Design review of the part built by this model. Coordinates are the model's own, in mm. A direction names the side the tool comes from. Round coordinates to 2 decimals unless told otherwise and drop trailing zeros. Loops run counter-clockwise (first coordinate to the right, second up) from the corner with the lowest first, then second, coordinate; pieces in that order, holes last. Notation, with made-up numbers: (63.5, 63) -> (72.5, 63) arc R11 ccw to (72.5, 76) -> close; hole circle Ø4 at (38.25, 79). An arc over 180 degrees is marked (long way). Answer as CSV lines item,"result". Start each with the question number.
(1) To check wall thickness, follow line 1 (Z direction, x = 45.5, y = -1.6); line 2 (Z direction, x = 25, y = -12); line 3 (X direction, y = -13, z = 18). State the ranges of each line that lie inside material, in increasing order. Write a range as from..to.
(2) Machinability: for faces 1 (the face through (6, -26, 44)), 2 (the face through (6, -26, 6)), 3 (the face through (43.254, -14.168, 6.485)), which of the approach directions +Z, -Z, +X, -X, +Y, -Y give a long, thin tool a straight path to every point of the face, cutting with its end or side? Answer none if there is none.
(3) Take a section at A-A, the plane z = 25. Write out the cut boundary in (x, y), and give its area (3 significant figures).
(4) Draft analysis for pull direction X (two halves, no side actions). For faces 4 (the face through (0, -14, 25)), 5 (the face through (43.515, -14.168, 43.254)), 6 (the face through (5.3, -1, 3)), 7 (the face through (25, -14, 50)), state which applies: +X half, -X half, draft (parallel to the pull), parting line (faces both ways), or undercut.
(5) Take a section at D-D, the plane x = 44.5. State how many separate pieces and enclosed holes the cut face has, and give its area (3 significant figures).
(6) Take a section at C-C, the plane y = -6.25. Write out the cut boundary in (x, z), and give its area (3 significant figures).
(7) Take a section at B-B, the plane x = 25. Write out the cut boundary in (y, z).
(8) For P1, Ø2.5, axis at x = 4.5, z = 4.5, coming from the -Y side; P2, Ø5.5, axis at x = 41.5, z = 38.5, coming from the -Y side; P3, Ø3, axis at x = 39.5, y = -23, coming from the -Z side, all flat-tipped, find the tip position at first contact; note any pin that passes through.
from build123d import *

# Parameters (mm, degrees)
SKETCH_W        = 50
SKETCH_H        = 50
PAD_DEPTH       = 28
SKETCH001_R     = 23
SKETCH001_R_2   = 1.7
POCKET_DEPTH    = 40
SKETCH002_W     = 75.459096
SKETCH002_H     = 67.94658
SKETCH002_R     = 26
POCKET001_DEPTH = 24


with BuildPart() as part:
    # Sketch → Pad (new body)
    with BuildSketch(Plane.XZ):
        with Locations((25, 25)):
            Rectangle(SKETCH_W, SKETCH_H)
    extrude(amount=PAD_DEPTH)

    # Sketch001 (on Face6 of Pad) → Pocket (cut)
    with BuildSketch(Plane.XZ.offset(28)):
        with Locations((25, 25)):
            Circle(SKETCH001_R)
        with Locations((4.5, 45.5)):
            Circle(SKETCH001_R_2)
        with Locations((4.5, 4.5)):
            Circle(SKETCH001_R_2)
        with Locations((45.5, 4.5)):
            Circle(SKETCH001_R_2)
        with Locations((45.5, 45.5)):
            Circle(SKETCH001_R_2)
    extrude(amount=-POCKET_DEPTH, mode=Mode.SUBTRACT)

    # Sketch002 (on DatumPlane) → Pocket001 (cut)
    with BuildSketch(Plane.XZ.offset(26)):
        with Locations((26.273557, 24.507667)):
            Rectangle(SKETCH002_W, SKETCH002_H)
        with Locations((25, 25)):
            Circle(SKETCH002_R, mode=Mode.SUBTRACT)
    extrude(amount=-POCKET001_DEPTH, mode=Mode.SUBTRACT)


solid = part.part
The answers:
1,line 1,"0..2.8, 6.2..14.57, 35.43..43.8, 47.2..50"
1,line 2,"0..2, 48..50"
1,line 3,"0..3.09, 46.91..50"
2,face 1,"+Z, -X"
2,face 2,"-Z, -X"
2,face 3,"-Z, +X"
3,outline,"(0, -28) -> (2, -28) -> (2, 0) -> (0, 0) -> close; (48, -28) -> (50, -28) -> (50, 0) -> (48, 0) -> close"
3,area,"112 mm²"
4,face 4,"-X half"
4,face 5,"+X half"
4,face 6,"undercut"
4,face 7,"draft"
5,separate pieces,"6"
5,enclosed holes,"0"
5,area,"320 mm²"
6,outline,"(0, 17.86) arc R26 ccw to (17.86, 0) -> (32.14, 0) arc R26 ccw to (50, 17.86) -> (50, 32.14) arc R26 ccw to (32.14, 50) -> (17.86, 50) arc R26 ccw to (0, 32.14) -> close; hole circle Ø46 at (25, 25)"
6,area,"424 mm²"
7,outline,"(-28, 0) -> (0, 0) -> (0, 2) -> (-28, 2) -> close; (-28, 48) -> (0, 48) -> (0, 50) -> (-28, 50) -> close"
8,P1,"through"
8,P2,"y = -28"
8,P3,"z = 2.48"
